For this review, take the finished solid that the model builds, in its own axes (mm). A direction names the side the tool comes from. Coordinates: 2 decimals unless noted, no trailing zeros. Write each loop counter-clockwise with the first axis right and the second up, starting at its lowest first coordinate (ties: lowest second). Pieces come first, ordered by that corner, then holes. Notation, with made-up numbers: (-21, -7) -> (26, -7) arc R28 cw to (26, 17) -> close; hole circle Ø11 at (33, 86.5). An arc over 180 degrees is marked (long way). One line per item, written item: value. Start each with the question number.
1) For pin 1 Ø4 at (x, y) = (15, -31.4) entering from +Z; pin 2 Ø1.2 at (y, z) = (-21.5, 3.5) entering from -X; pin 3 Ø2 at (x, z) = (-7, 2.5) entering from +Y; pin 4 Ø2 at (y, z) = (16, 0.5) entering from -X, all flat-tipped, find the tip position at first contact; note any pin that passes through.
2) Add section C-C (y = -27). State the section outline as (x, z) points, and give its area (3 significant figures).
3) Machinability: for faces 4 (the cylindrical face through (84.218, -11.665, 2.535)), 5 (the flat face through (5, -32, 2)), 6 (the flat face through (45, -19.4, 2)), which of the approach directions +Z, -Z, +X, -X, +Y, -Y give a long, thin tool a straight path to every point of the face, cutting with its end or side? Answer none if there is none.
4) Add section D-D (x = 23). State the section outline as (y, z) points, and give its area (3 significant figures).
5) Add section B-B (z = 3.05). State how many separate pieces and enclosed holes the cut face has, and give its area (3 significant figures).
6) Add section A-A (x = 75). State the section outline as (y, z) points, and give its area (3 significant figures).
7) Mouldability with a two-part tool opening along Y and no side actions: class faces 1 (the flat face through (27, 3, 5)), 2 (the cylindrical face through (14.67, -43.87, 2.54)), 3 (the cylindrical face through (4.218, -11.665, 2.535)) as released by +Y, released by -Y, zero draft, split by the parting line, or undercut.
8) For probe 1 along Y at (x, z) = (0, 2.4); probe 2 along Y at (x, z) = (75, 2.75); probe 3 along Y at (x, z) = (14, 4.5), list the stretches that pass through material, from the lowest coordinate up. Write a range as from..to.
from build123d import *

# Parameters (mm, degrees)
SKETCH_1_R          = 2.55
SKETCH_1_R_2        = 8.4
EXTRUDE_1_DEPTH     = 5
FILLET_1_R          = 10
SKETCH_2_R          = 2.55
CUT_EXTRUDE_1_DEPTH = 112.121375081
FILLET_2_R          = 30
SKETCH_3_W          = 40
SKETCH_3_H          = 3
CUT_EXTRUDE_2_DEPTH = 112.121375081
SKETCH_5_W          = 40
SKETCH_5_H          = 0.5
CUT_EXTRUDE_4_DEPTH = 112.121375081
FILLET_3_R          = 1
CUT_EXTRUDE_5_DEPTH = 112.121375081
FILLET_4_R          = 5
SKETCH_7_R          = 1.25
CUT_EXTRUDE_6_DEPTH = 110.538877646


with BuildPart() as part:
    # ｽｹｯﾁ1 → ﾎﾞｽ - 押し出し1 (new body)
    with BuildSketch(Plane.XY):
        with BuildLine():
            Line((40, 33.6), (85, -11.4))
            Line((85, -11.4), (85, -71.4))
            Line((85, -71.4), (5, -71.4))
            Line((5, -71.4), (5, -11.4))
            Line((5, -11.4), (-40, 33.6))
            ThreePointArc((-40, 33.6), (0, 68.911288741), (40, 33.6))
        make_face()
        with Locations((75, -31.4)):
            Circle(SKETCH_1_R, mode=Mode.SUBTRACT)
        with Locations((75, -56.4)):
            Circle(SKETCH_1_R, mode=Mode.SUBTRACT)
        with Locations((0, 23.6)):
            Circle(SKETCH_1_R, mode=Mode.SUBTRACT)
        with Locations((0, 48.6)):
            Circle(SKETCH_1_R_2, mode=Mode.SUBTRACT)
    extrude(amount=EXTRUDE_1_DEPTH)

    # ﾌｨﾚｯﾄ1
    fillet_1_edges = [part.edges().sort_by_distance(p)[0] for p in [
        (40, 33.6, 2.5),
        (85, -11.4, 2.5),
        (5, -11.4, 2.5),
    ]]
    fillet(fillet_1_edges, radius=FILLET_1_R)

    # ｽｹｯﾁ2 → ｶｯﾄ - 押し出し1 (cut, through all)
    with BuildSketch(Plane.XY.offset(5)):
        with Locations((15, -46.4)):
            Circle(SKETCH_2_R)
        with Locations((15, -31.4)):
            Circle(SKETCH_2_R)
    extrude(amount=-CUT_EXTRUDE_1_DEPTH, mode=Mode.SUBTRACT)

    # ﾌｨﾚｯﾄ2
    fillet_2_edges = [part.edges().sort_by_distance(p)[0] for p in [
        (-40, 33.6, 2.5),
    ]]
    fillet(fillet_2_edges, radius=FILLET_2_R)

    # ｽｹｯﾁ3 → ｶｯﾄ - 押し出し2 (cut, through all)
    with BuildSketch(Plane(origin=(0, 0, 0), x_dir=(-1, 0, 0), z_dir=(0, 0, -1))):
        with Locations((-45, -21.4)):
            Rectangle(SKETCH_3_W, SKETCH_3_H)
    extrude(amount=-CUT_EXTRUDE_2_DEPTH, mode=Mode.SUBTRACT)

    # ｽｹｯﾁ5 → ｶｯﾄ - 押し出し4 (cut, through all)
    with BuildSketch(Plane(origin=(0, 0, 0), x_dir=(-1, 0, 0), z_dir=(0, 0, -1))):
        with Locations((-45, -19.65)):
            Rectangle(SKETCH_5_W, SKETCH_5_H)
    extrude(amount=-CUT_EXTRUDE_4_DEPTH, mode=Mode.SUBTRACT)

    # ﾌｨﾚｯﾄ3
    fillet_3_edges = [part.edges().sort_by_distance(p)[0] for p in [
        (25, -22.9, 2.5),
        (65, -22.9, 2.5),
        (65, -19.4, 2.5),
        (25, -19.4, 2.5),
    ]]
    fillet(fillet_3_edges, radius=FILLET_3_R)

    # ｽｹｯﾁ6 → ｶｯﾄ - 押し出し5 (cut, through all)
    with BuildSketch(Plane(origin=(0, 0, 0), x_dir=(-1, 0, 0), z_dir=(0, 0, -1))):
        Polygon((-5, -51.829889619), (-122.420662288, -71.4), (-5, -71.4), align=None)
    extrude(amount=-CUT_EXTRUDE_5_DEPTH, mode=Mode.SUBTRACT)

    # ﾌｨﾚｯﾄ4
    fillet_4_edges = [part.edges().sort_by_distance(p)[0] for p in [
        (85, -65.163222952, 2.5),
        (5, -51.829889619, 2.5),
    ]]
    fillet(fillet_4_edges, radius=FILLET_4_R)

    # ｽｹｯﾁ7 → ｶｯﾄ - 押し出し6 (cut, through all)
    with BuildSketch(Plane.XY.offset(5)):
        with Locations((0, 63.6)):
            Circle(SKETCH_7_R)
        with Locations((15, 48.6)):
            Circle(SKETCH_7_R)
        with Locations((0, 33.6)):
            Circle(SKETCH_7_R)
        with Locations((-15, 48.6)):
            Circle(SKETCH_7_R)
    extrude(amount=-CUT_EXTRUDE_6_DEPTH, mode=Mode.SUBTRACT)


solid = part.part
Numbers:
1. pin 1: through
1. pin 2: x = 5
1. pin 3: y = 68.46
1. pin 4: x = -23.4
2. outline: (5, 0) -> (85, 0) -> (85, 5) -> (5, 5) -> close
2. area: 400 mm²
3. face 4: +Z, -Z, +X, +Y
3. face 5: +Z, -Z, -X, -Y
3. face 6: +Z, -Z
4. outline: (-54.83, 0) -> (61.71, 0) -> (61.71, 5) -> (-54.83, 5) -> close
4. area: 583 mm²
5. separate pieces: 1
5. enclosed holes: 11
5. area: 8,850 mm²
6. outline: (-63.5, 0) -> (-58.95, 0) -> (-58.95, 5) -> (-63.5, 5) -> close; (-53.85, 0) -> (-33.95, 0) -> (-33.95, 5) -> (-53.85, 5) -> close; (-28.85, 0) -> (-1.4, 0) -> (-1.4, 5) -> (-28.85, 5) -> close
6. area: 259 mm²
7. face 1: zero draft
7. face 2: undercut
7. face 3: released by -Y
8. probe 1: -6.4..21.05, 26.15..32.35, 34.85..40.2, 57..62.35, 64.85..68.91
8. probe 2: -63.5..-58.95, -53.85..-33.95, -28.85..-1.4
8. probe 3: -53.33..-48.75, -44.05..-33.75, -29.05..47.85, 49.35..66.4
